from build123d import *

# Parameters (mm, degrees)
SKETCH1_R                                       = 14.2875
BOSS_EXTRUDE1_DEPTH                             = 6.35
F_3_4_0_75_DIAMETER_HOLE1_D                     = 19.05
CBORE_FOR_10_BUTTON_HEAD_CAP_SCREW1_D           = 5.1054
CBORE_FOR_10_BUTTON_HEAD_CAP_SCREW1_CBORE_D     = 9.92124
CBORE_FOR_10_BUTTON_HEAD_CAP_SCREW1_CBORE_DEPTH = 2.5654
F_1_4_CLEARANCE_HOLE1_D                         = 6.7564
F_10_CLEARANCE_HOLE2_D                          = 5.1054
CUT_EXTRUDE2_DEPTH                              = 3.175
CUT_EXTRUDE3_DEPTH                              = 182.28977969


with BuildPart() as part:
    # Sketch1 → Boss-Extrude1 (new body)
    with BuildSketch(Plane.XY):
        with BuildLine():
            Line((-120.65, 0), (-117.17933671, 0))
            ThreePointArc((-117.17933671, 0), (-115.59183671, 1.5875), (-114.00433671, 0))
            Line((-114.00433671, 0), (-114.00433671, -4.7625))
            Line((-114.00433671, -4.7625), (-104.47933671, -4.7625))
            ThreePointArc((-104.47933671, -4.7625), (-102.234272679, -5.69243597), (-101.30433671, -7.9375))
            Line((-101.30433671, -7.9375), (-101.30433671, -9.525))
            Line((-101.30433671, -9.525), (-60.02933671, -9.525))
            Line((-60.02933671, -9.525), (-60.02933671, 0))
            ThreePointArc((-60.02933671, 0), (-58.44183671, 1.5875), (-56.85433671, 0))
            Line((-56.85433671, 0), (-38.1, 0))
            ThreePointArc((-38.1, 0), (-30.815579258, 2.296769038), (-26.165903716, 8.35634418))
            Line((-26.165903716, 8.35634418), (-20.945967504, 22.698001054))
            ThreePointArc((-20.945967504, 22.698001054), (-17.273923344, 27.999473263), (-11.471463484, 30.813896024))
            ThreePointArc((-11.471463484, 30.813896024), (-7.639410119, 33.209590086), (-6.371263462, 37.547306891))
            ThreePointArc((-6.371263462, 37.547306891), (-2.360982527, 57.822228263), (11.645315486, 73.020202003))
            ThreePointArc((11.645315486, 73.020202003), (21.385338266, 98.001275259), (0, 114.175))
            ThreePointArc((0, 114.175), (-27.81071387, 117.557961662), (-53.999382782, 127.509537225))
            ThreePointArc((-53.999382782, 127.509537225), (-65.649094725, 128.437962549), (-74.359242294, 120.64623031))
            Line((-74.359242294, 120.64623031), (-126.405054448, 9.033625962))
            ThreePointArc((-126.405054448, 9.033625962), (-126.005535681, 2.938147487), (-120.65, 0))
        make_face()
        with Locations((0, 91.95)):
            Circle(SKETCH1_R, mode=Mode.SUBTRACT)
    extrude(amount=BOSS_EXTRUDE1_DEPTH)

    # 3/4 (0.75) Diameter Hole1 (through all)
    with Locations(Plane.XY.offset(6.35)):
        with Locations((-49.493351826, 63.375)):
            Hole(F_3_4_0_75_DIAMETER_HOLE1_D / 2)

    # CBORE for #10 Button Head Cap Screw1 (through all)
    with Locations(Plane(origin=(0, 0, 6.35), x_dir=(-1, 0, 0), z_dir=(0, 0, 1))):
        with Locations((24.093351826, -63.375), (74.893351826, -63.375)):
            CounterBoreHole(CBORE_FOR_10_BUTTON_HEAD_CAP_SCREW1_D / 2, CBORE_FOR_10_BUTTON_HEAD_CAP_SCREW1_CBORE_D / 2, CBORE_FOR_10_BUTTON_HEAD_CAP_SCREW1_CBORE_DEPTH)

    # 1/4 Clearance Hole1 (through all)
    with Locations(Plane(origin=(0, 0, 0), x_dir=(-1, 0, 0), z_dir=(0, 0, -1))):
        with Locations((67.96683671, 6.35), (106.06683671, 6.35)):
            Hole(F_1_4_CLEARANCE_HOLE1_D / 2)

    # #10 Clearance Hole2 (through all)
    with Locations(Plane(origin=(0, 0, 0), x_dir=(-1, 0, 0), z_dir=(0, 0, -1))):
        with Locations((60.908084373, 114.37385236), (12.701259616, 37.043671419)):
            Hole(F_10_CLEARANCE_HOLE2_D / 2)

    # Sketch20 → Cut-Extrude2 (cut, symmetric)
    with BuildSketch(Plane(origin=(0, 0, 6.35), x_dir=(-1, 0, 0), z_dir=(0, 0, -1))):
        with BuildLine():
            Line((92.44330918, 48.057718602), (98.198363628, 50.741344564))
            ThreePointArc((98.198363628, 50.741344564), (100.30803373, 49.973487442), (99.540176609, 47.86381734))
            Line((99.540176609, 47.86381734), (110.274680457, 24.843599549))
            ThreePointArc((110.274680457, 24.843599549), (112.384350559, 24.075742428), (111.616493438, 21.966072325))
            Line((111.616493438, 21.966072325), (105.86143899, 19.282446363))
            ThreePointArc((105.86143899, 19.282446363), (103.751768888, 20.050303485), (104.519626009, 22.159973587))
            Line((104.519626009, 22.159973587), (93.785122161, 45.180191378))
            ThreePointArc((93.785122161, 45.180191378), (91.675452059, 45.948048499), (92.44330918, 48.057718602))
        make_face()
        with BuildLine():
            Line((70.34966907, 110.463062771), (72.362388541, 106.146771935))
            ThreePointArc((72.362388541, 106.146771935), (74.525057067, 104.165051345), (71.59453142, 104.037101832))
            Line((71.59453142, 104.037101832), (68.717004196, 102.695288851))
            ThreePointArc((68.717004196, 102.695288851), (66.735283607, 100.532620325), (66.607334094, 103.463145973))
            Line((66.607334094, 103.463145973), (65.265521113, 106.340673197))
            ThreePointArc((65.265521113, 106.340673197), (63.15585101, 107.108530318), (63.923708132, 109.21820042))
            Line((63.923708132, 109.21820042), (68.239998967, 111.230919892))
            ThreePointArc((68.239998967, 111.230919892), (70.221719557, 113.393588418), (70.34966907, 110.463062771))
        make_face()
    extrude(amount=CUT_EXTRUDE2_DEPTH, both=True, mode=Mode.SUBTRACT)

    # Sketch21 → Cut-Extrude3 (cut, through all)
    with BuildSketch(Plane(origin=(0, 0, 0), x_dir=(-1, 0, 0), z_dir=(0, 0, -1))):
        with BuildLine():
            Line((94.995724075, 20.045977116), (85.987083429, 39.365069327))
            ThreePointArc((85.987083429, 39.365069327), (79.023116956, 44.717335237), (70.640334696, 42.095782075))
            ThreePointArc((70.640334696, 42.095782075), (68.891484629, 40.490235554), (67.021153622, 39.028005027))
            ThreePointArc((67.021153622, 39.028005027), (64.697142252, 35.852583725), (64.690284199, 31.917576449))
            Line((64.690284199, 31.917576449), (67.728953723, 22.537639163))
            ThreePointArc((67.728953723, 22.537639163), (69.288161522, 19.996093098), (71.835528588, 18.446413648))
            ThreePointArc((71.835528588, 18.446413648), (76.138470899, 16.071851402), (79.217676493, 12.241400867))
            ThreePointArc((79.217676493, 12.241400867), (90.920159406, 8.434245512), (94.995724075, 20.045977116))
        make_face()
        with BuildLine():
            Line((51.469052768, 9.525), (44.769476801, 9.525))
            ThreePointArc((44.769476801, 9.525), (37.48505606, 11.821769038), (32.835380517, 17.88134418))
            Line((32.835380517, 17.88134418), (29.231939453, 27.781717136))
            ThreePointArc((29.231939453, 27.781717136), (30.834227059, 34.565634102), (37.696077358, 35.791956022))
            ThreePointArc((37.696077358, 35.791956022), (41.894327789, 34.353373001), (46.258868743, 33.549874364))
            ThreePointArc((46.258868743, 33.549874364), (52.902583174, 30.776932908), (56.971445845, 24.83786713))
            Line((56.971445845, 24.83786713), (58.667572518, 19.6021672))
            ThreePointArc((58.667572518, 19.6021672), (58.894836065, 16.629132278), (57.740046713, 13.880123927))
            ThreePointArc((57.740046713, 13.880123927), (57.33778938, 13.300780738), (56.968314082, 12.7))
            ThreePointArc((56.968314082, 12.7), (54.644052768, 10.375738686), (51.469052768, 9.525))
        make_face()
        with BuildLine():
            ThreePointArc((46.049330406, 93.17665627), (39.806875451, 91.768171282), (34.005177492, 89.067731575))
            ThreePointArc((34.005177492, 89.067731575), (26.46144828, 88.715057819), (22.036931884, 94.835179049))
            ThreePointArc((22.036931884, 94.835179049), (21.648773671, 96.978043711), (21.052760506, 99.072632947))
            ThreePointArc((21.052760506, 99.072632947), (21.553789247, 104.256924834), (25.764522177, 107.322481938))
            ThreePointArc((25.764522177, 107.322481938), (33.843976098, 109.298383447), (41.774843757, 111.804994829))
            ThreePointArc((41.774843757, 111.804994829), (46.260154558, 111.70723207), (49.56139318, 108.669240282))
            ThreePointArc((49.56139318, 108.669240282), (50.30920774, 107.37715213), (51.203478444, 106.181744954))
            ThreePointArc((51.203478444, 106.181744954), (52.517215708, 98.137202873), (46.049330406, 93.17665627))
        make_face()
    extrude(amount=-CUT_EXTRUDE3_DEPTH, mode=Mode.SUBTRACT)


solid = part.part
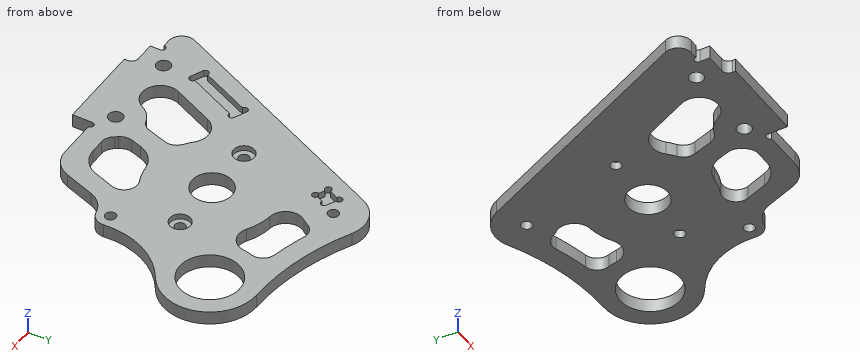
Geometry check sheet. Reference: the model listing, model coordinates, mm. Give positions to 0.01 mm unless a question says otherwise; leave off trailing zeros. Write each loop counter-clockwise with the first axis right and the second up, starting at its lowest first coordinate (ties: lowest second). Pieces come first, ordered by that corner, then holes. Notation, with made-up numbers: (5, -17) - (39, -17) arc R12 ccw to (39, 3) - close; hole circle Ø10 at (-38, -25.75). An arc over 180 degrees is marked (long way). Put each result on its own line as item: value.
1. Go/stop test with flat-tipped pins: pin 1 (1.4 mm diameter, centred on y = -2, z = 1.5, fed in from -X); pin 2 (1.9 mm diameter, centred on x = -108, z = 3, fed in from -Y); pin 3 (3 mm diameter, centred on x = -101.5, z = 3.5, fed in from +Y); pin 4 (17 mm diameter, centred on x = 0, y = 91.95, fed in from +Z). Record where each tip stops, or that it passes through.
Ans:
pin 1: stops at x = -114
pin 2: stops at y = -4.76
pin 3: stops at y = 65.66
pin 4: passes through
2. Sectioned sample at B-B, the plane z = 1. Give the number of separate pieces and of enclosed holes in the cut face, plus the area to 3 significant figures.
Ans:
separate pieces: 1
enclosed holes: 11
area: 9,740 mm²
3. Sectioned sample at A-A, the plane y = 79.5. Enter the section's corners in (x, z), plus the area to 3 significant figures.
Ans:
outline: (-93.55, 0) - (-7.01, 0) - (-7.01, 6.35) - (-93.55, 6.35) - close; (7.01, 0) - (18.41, 0) - (18.41, 6.35) - (7.01, 6.35) - close
area: 622 mm²
4. Thickness scan on line 1 (X direction, y = 24, z = 4.5); line 2 (Y direction, x = -33.5, z = 3.5); line 3 (X direction, y = 4.5, z = 3.5). Record the ranges inside material, lowest first.
Ans:
line 1: x = -119.43 to -112.42, -103.66 to -93.15, -67.26 to -57.24, -30.61 to -20.39
line 2: y = 0.86 to 16.37, 36.07 to 88.79, 109.2 to 119.12
line 3: x = -126.72 to -108.89, -103.24 to -70.79, -65.14 to -28.4
